CAD build for the part. Positions are in the model's coordinates, mm. Give positions to 0.01 mm unless a question says otherwise; leave off trailing zeros. Write each loop counter-clockwise with the first axis right and the second up, starting at its lowest first coordinate (ties: lowest second). Pieces come first, ordered by that corner, then holes. Notation, with made-up numbers: M 20,-35 L 58,-35 A14 cw 58,-24 Z; hole C 7.25,80 d3. An arc over 180 degrees is marked long. One line per question, with ' | ' between items. Start each with the question number.
1. Wall check: L1, parallel to Z at x = 5.5, y = 13. Give the ranges that are in metal, low to high.
2. Flat gauge pin, fed straight in: pin 1 (13.5 mm diameter, centred on x = 7, y = -6.5, fed in from +Z). Where does the tip first touch, or does it go through?
3. Cut at A-A, the plane z = 20.75. Write the cut outline in (x, y).
4. Cut at C-C, the plane x = 17. Write the cut outline in (y, z), then the cut area to 3 significant figures.
5. Cut at B-B, the plane y = -6. Write the cut outline in (x, z).
```python
from build123d import *

# Parameters (mm, degrees)
SKETCH_1_W      = 50
SKETCH_1_H      = 45
EXTRUDE_1_DEPTH = 20
SKETCH_2_R      = 0.5
EXTRUDE_2_DEPTH = 5


with BuildPart() as part:
    # Эскиз1 → Вытянуть1 (new body)
    with BuildSketch(Plane.XY):
        Rectangle(SKETCH_1_W, SKETCH_1_H)
    extrude(amount=EXTRUDE_1_DEPTH)

    # Эскиз2 → Вытянуть2 (add)
    with BuildSketch(Plane.XY.offset(20)):
        with Locations(Location((-21.5, 17.5, 0), (0, 0, 180))):
            Circle(SKETCH_2_R)
        with Locations(Location((-21.5, 0, 0), (0, 0, 180))):
            Circle(SKETCH_2_R)
        with Locations(Location((21.5, 0, 0), (0, 0, 180))):
            Circle(SKETCH_2_R)
        with Locations(Location((21.5, 10, 0), (0, 0, 180))):
            Circle(SKETCH_2_R)
        with Locations(Location((21.5, -10, 0), (0, 0, 180))):
            Circle(SKETCH_2_R)
    extrude(amount=EXTRUDE_2_DEPTH)


solid = part.part
```
Here are the results:
1) L1: 0 to 20
2) pin 1: z = 20
3) outline: C -21.5,0 d1; C -21.5,17.5 d1; C 21.5,-10 d1; C 21.5,0 d1; C 21.5,10 d1
4) outline: M -22.5,0 L 22.5,0 L 22.5,20 L -22.5,20 Z | area: 900 mm^2
5) outline: M -25,0 L 25,0 L 25,20 L -25,20 Z
